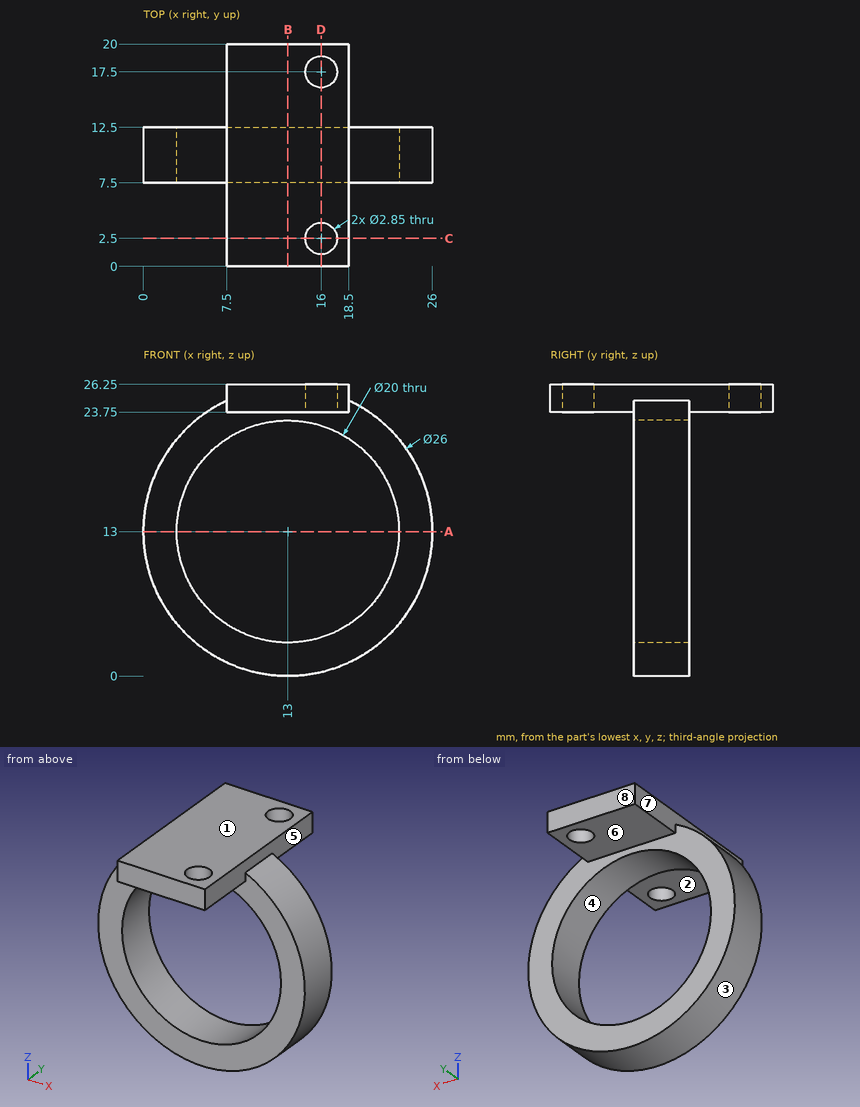
Could you check a few things on this drawing? It's one solid part, dimensions in mm from its lowest x, y, z. A direction names the side the tool comes from. Coordinates: 2 decimals unless noted, no trailing zeros. Write each loop counter-clockwise with the first axis right and the second up, starting at its lowest first coordinate (ties: lowest second). Pieces come first, ordered by that corner, then holes.
1) If we section it at C-C (y = 2.5): List the corners of the cut face in (x, z) for me (3 decimals), plus the area to 3 significant figures.
Filled in:
outline: (7.5, 23.75) - (14.575, 23.75) - (14.575, 26.25) - (7.5, 26.25) - close; (17.425, 23.75) - (18.5, 23.75) - (18.5, 26.25) - (17.425, 26.25) - close
area: 20.4 mm2
2) If I drill on line 1 (Y direction, x = 16, z = 24.9) (3 decimals); line 2 (Z direction, x = 13, y = 9.9); line 3 (X direction, y = 2.5, z = 24.35) (3 decimals), over which ranges is the centre line in solid material (lowest first)?
Filled in:
line 1: y = 0 to 1.075, 3.925 to 16.075, 18.925 to 20
line 2: z = 0 to 3, 23 to 26.25
line 3: x = 7.5 to 14.575, 17.425 to 18.5
3) If we section it at B-B (x = 13): List the corners of the cut face in (y, z) for me, plus the area to 4 significant figures.
Filled in:
outline: (0, 23.75) - (7.5, 23.75) - (7.5, 23) - (12.5, 23) - (12.5, 23.75) - (20, 23.75) - (20, 26.25) - (0, 26.25) - close; (7.5, 0) - (12.5, 0) - (12.5, 3) - (7.5, 3) - close
area: 68.75 mm2
4) Thinking about a two-plate mould opening in Z: for the marked faces 1, 2, 3 and 4, which applies, +Z half, -Z half, draft (parallel to the pull), parting line (faces both ways), or undercut?
Filled in:
face 1: +Z half
face 2: -Z half
face 3: parting line
face 4: undercut
5) If we section it at A-A (z = 13): List the corners of the cut face in (x, y) for me, plus the area to 3 significant figures.
Filled in:
outline: (0, 7.5) - (3, 7.5) - (3, 12.5) - (0, 12.5) - close; (23, 7.5) - (26, 7.5) - (26, 12.5) - (23, 12.5) - close
area: 30.0 mm2
6) Which directions (+Z, -Z, +X, -X, +Y, -Y) give clear straight access to the entire face, cutting with the end or side of a thin tool? Please do the marked faces 5, 6, 7 and 8.
Filled in:
face 5: +Z, +X
face 6: -Z, +X, -X, +Y
face 7: +Z, -X
face 8: +Z, -Z, +X, -X, +Y
7) If we section it at D-D (x = 16): List the corners of the cut face in (y, z) for me (3 decimals), plus the area to 3 significant figures.
Filled in:
outline: (0, 23.75) - (1.075, 23.75) - (1.075, 26.25) - (0, 26.25) - close; (3.925, 23.75) - (7.5, 23.75) - (7.5, 22.539) - (12.5, 22.539) - (12.5, 23.75) - (16.075, 23.75) - (16.075, 26.25) - (3.925, 26.25) - close; (7.5, 0.351) - (12.5, 0.351) - (12.5, 3.461) - (7.5, 3.461) - close; (18.925, 23.75) - (20, 23.75) - (20, 26.25) - (18.925, 26.25) - close
area: 57.4 mm2
8) I'm going to push flat-ended pins straight in: pin 1 (1.2 mm diameter, centred on y = 6.5, z = 25, fed in from -X); pin 2 (3 mm diameter, centred on x = 3, z = 10.5, fed in from -Y); pin 3 (8 mm diameter, centred on x = 12, y = 4.5, fed in from -Z); pin 4 (3.5 mm diameter, centred on x = 16, y = 17.5, fed in from -Z). Where does each tip first touch, or does it pass through?
Filled in:
pin 1: stops at x = 7.5
pin 2: stops at y = 7.5
pin 3: stops at z = 0
pin 4: stops at z = 23.75
